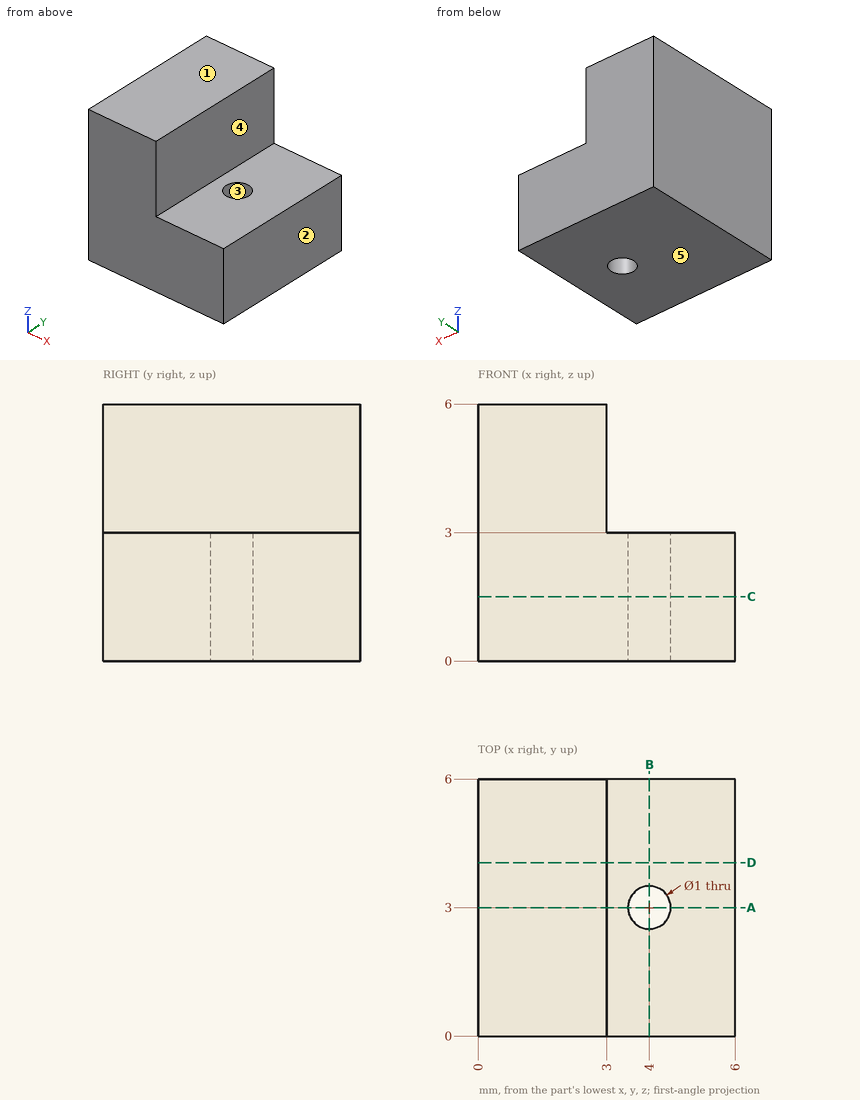
Study the drawing (mm; zero at the part's minimum x, y, z) and answer. A direction names the side the tool comes from. Coordinates: 2 decimals unless noted, no trailing zeros. Loops run counter-clockwise (first coordinate to the right, second up) from the corner with the lowest first, then second, coordinate; pieces in that order, holes last. Notation, with made-up numbers: (-23, -30.5) -> (21, -30.5) arc R14 cw to (21, -26.5) -> close; hole circle Ø4 at (13.25, 66.25). An arc over 180 degrees is marked (long way). Write each question's results on one line, items separated by ' | '. Start each with the question number.
1) For the marked faces 4 and 5, determine the directions among +Z, -Z, +X, -X, +Y, -Y from which every point of the face is accessible in a straight line to the end or side of a thin tool.
2) Find section C-C on z = 1.5. Determine the outline of the cut face in (x, y), then the cut area to 3 significant figures.
3) The mould has two halves that part along X. Classify the marked faces 1, 2 and 3: pulls with the +X half, pulls with the -X half, needs draft (parallel to the pull), parting line crosses it, or undercut.
4) Find section D-D on y = 4.05. Determine the outline of the cut face in (x, z).
5) Flat-ended cylindrical pins translate along their axes: P1, Ø0.9, axis at y = 2.5, z = 5, coming from the +X side; P2, Ø0.9, axis at x = 4, y = 4, coming from the +Z side. Find the tip coordinate at first contact, or state that the pin passes through.
6) Find section A-A on y = 3. Determine the outline of the cut face in (x, z).
7) Consider line 1 along Y through (x, z) = (4, 2.05); line 2 along Z through (x, y) = (4.55, 1.4). Determine where each line is inside the solid, lowest interval first.
8) Find section B-B on x = 4. Determine the outline of the cut face in (y, z), then the cut area to 3 significant figures.
Response values:
1) face 4: +Z, +X, +Y, -Y | face 5: -Z, +X, -X, +Y, -Y
2) outline: (0, 0) -> (6, 0) -> (6, 6) -> (0, 6) -> close; hole circle Ø1 at (4, 3) | area: 35.2 mm^2
3) face 1: needs draft | face 2: pulls with the +X half | face 3: undercut
4) outline: (0, 0) -> (6, 0) -> (6, 3) -> (3, 3) -> (3, 6) -> (0, 6) -> close
5) P1: stops at x = 3 | P2: stops at z = 3
6) outline: (0, 0) -> (3.5, 0) -> (3.5, 3) -> (3, 3) -> (3, 6) -> (0, 6) -> close; (4.5, 0) -> (6, 0) -> (6, 3) -> (4.5, 3) -> close
7) line 1: y = 0 to 2.5, 3.5 to 6 | line 2: z = 0 to 3
8) outline: (0, 0) -> (2.5, 0) -> (2.5, 3) -> (0, 3) -> close; (3.5, 0) -> (6, 0) -> (6, 3) -> (3.5, 3) -> close | area: 15.0 mm^2
